from build123d import *

# Parameters (mm, degrees)
SKETCH1_W                = 90
SKETCH1_H                = 90
BOSS_EXTRUDE1_DEPTH      = 90
SKETCH4_W                = 40
SKETCH4_H                = 80
CUT_EXTRUDE3_DEPTH       = 90
SKETCH6_W                = 10
SKETCH6_H                = 2.5
CUT_EXTRUDE5_DEPTH       = 10
CUT_EXTRUDE6_DEPTH       = 90
CUT_EXTRUDE7_DEPTH       = 90
SKETCH10_W               = 2.5
SKETCH10_H               = 90
BOSS_EXTRUDE2_DEPTH      = 40
SKETCH11_W               = 2.5
SKETCH11_H               = 90
BOSS_EXTRUDE3_DEPTH      = 40
CUT_EXTRUDE10_DEPTH      = 37.5
SKETCH16_R               = 0.75
CUT_EXTRUDE12_DEPTH      = 1.5
CUT_EXTRUDE13_DEPTH      = 111.227038425
CUT_EXTRUDE13_DEPTH_BACK = 111.227038425
SKETCH17_R               = 0.75
SKETCH21_W               = 85
SKETCH21_H               = 2.5
CUT_EXTRUDE14_DEPTH      = 40
SKETCH22_W               = 85
SKETCH22_H               = 2.5
CUT_EXTRUDE15_DEPTH      = 40
SKETCH23_R               = 1.25
CUT_EXTRUDE16_DEPTH      = 1.5
SKETCH24_R               = 1.25
CUT_EXTRUDE17_DEPTH      = 1.5


with BuildPart() as part:
    # Sketch1 → Boss-Extrude1 (new body)
    with BuildSketch(Plane(origin=(0, 0, 0), x_dir=(1, 0, 0), z_dir=(0, 1, 0))):
        Rectangle(SKETCH1_W, SKETCH1_H)
    extrude(amount=BOSS_EXTRUDE1_DEPTH)

    # Sketch4 → Cut-Extrude3 (cut)
    with BuildSketch(Plane(origin=(0, 90, 0), x_dir=(1, 0, 0), z_dir=(0, 1, 0))):
        with Locations((-22.5, 0)):
            Rectangle(SKETCH4_W, SKETCH4_H)
        with Locations((22.5, 0)):
            Rectangle(SKETCH4_W, SKETCH4_H)
    extrude(amount=-CUT_EXTRUDE3_DEPTH, mode=Mode.SUBTRACT)

    # Sketch6 → Cut-Extrude5 (cut)
    with BuildSketch(Plane.XY.offset(45)):
        with Locations((7.5, 1.25)):
            Rectangle(SKETCH6_W, SKETCH6_H)
        with Locations((-7.5, 1.25)):
            Rectangle(SKETCH6_W, SKETCH6_H)
    extrude(amount=-CUT_EXTRUDE5_DEPTH, mode=Mode.SUBTRACT)

    # Sketch7 → Cut-Extrude6 (cut)
    with BuildSketch(Plane(origin=(0, 90, 0), x_dir=(1, 0, 0), z_dir=(0, 1, 0))):
        Polygon((42.5, 40), (42.5, 45), (45, 45), (45, -45), (42.5, -45), (42.5, -40), align=None)
    extrude(amount=-CUT_EXTRUDE6_DEPTH, mode=Mode.SUBTRACT)

    # Sketch8 → Cut-Extrude7 (cut)
    with BuildSketch(Plane(origin=(0, 90, 0), x_dir=(1, 0, 0), z_dir=(0, 1, 0))):
        Polygon((-42.5, 40), (-42.5, 45), (-45, 45), (-45, -45), (-42.5, -45), (-42.5, -42.5), align=None)
    extrude(amount=-CUT_EXTRUDE7_DEPTH, mode=Mode.SUBTRACT)

    # Sketch10 → Boss-Extrude2 (add)
    with BuildSketch(Plane.ZY.offset(2.5)):
        with Locations((-28.75, 45)):
            Rectangle(SKETCH10_W, SKETCH10_H)
    extrude(amount=BOSS_EXTRUDE2_DEPTH)

    # Sketch11 → Boss-Extrude3 (add)
    with BuildSketch(Plane(origin=(2.5, 0, 0), x_dir=(0, 0, -1), z_dir=(1, 0, 0))):
        with Locations((28.75, 45)):
            Rectangle(SKETCH11_W, SKETCH11_H)
    extrude(amount=BOSS_EXTRUDE3_DEPTH)

    # Sketch13 → Cut-Extrude10 (cut)
    with BuildSketch(Plane(origin=(42.5, 0, 0), x_dir=(0, 0, -1), z_dir=(1, 0, 0))):
        Polygon((40, 36), (40.5, 36), (40.5, 37), (41, 37), (41, 35), (40, 35), align=None)
        Polygon((29, 35), (30, 35), (30, 36), (29.5, 36), (29.5, 37), (29, 37), align=None)
    cut_extrude10 = extrude(amount=-CUT_EXTRUDE10_DEPTH, mode=Mode.SUBTRACT)

    # Mirror1: Cut-Extrude10 across plane
    add(cut_extrude10.mirror(Plane.ZY), mode=Mode.SUBTRACT)

    # Sketch16 → Cut-Extrude12 (cut)
    with BuildSketch(Plane(origin=(-12.5, 0, 0), x_dir=(0, 0, -1), z_dir=(1, 0, 0))):
        with Locations((-43.75, 1.2)):
            Circle(SKETCH16_R)
    extrude(amount=-CUT_EXTRUDE12_DEPTH, mode=Mode.SUBTRACT)

    # Sketch17 → Cut-Extrude13 (cut, two sides: drawn at the far end of the back side and taken through both)
    with BuildSketch(Plane.ZY.offset(2.5).offset(-CUT_EXTRUDE13_DEPTH_BACK)):
        with Locations(Location((43.75, 1.2, 0), (0, 0, 180))):
            Circle(SKETCH17_R)
    extrude(amount=CUT_EXTRUDE13_DEPTH + CUT_EXTRUDE13_DEPTH_BACK, mode=Mode.SUBTRACT)

    # Sketch21 → Cut-Extrude14 (cut)
    with BuildSketch(Plane(origin=(42.5, 0, 0), x_dir=(0, 0, -1), z_dir=(1, 0, 0))):
        with Locations((2.5, 1.25)):
            Rectangle(SKETCH21_W, SKETCH21_H)
    extrude(amount=-CUT_EXTRUDE14_DEPTH, mode=Mode.SUBTRACT)

    # Sketch22 → Cut-Extrude15 (cut)
    with BuildSketch(Plane.ZY.offset(42.5)):
        with Locations((-2.5, 1.25)):
            Rectangle(SKETCH22_W, SKETCH22_H)
    extrude(amount=-CUT_EXTRUDE15_DEPTH, mode=Mode.SUBTRACT)

    # Sketch23 → Cut-Extrude16 (cut)
    with BuildSketch(Plane(origin=(42.5, 0, 0), x_dir=(0, 0, -1), z_dir=(1, 0, 0))):
        with Locations((42.5, 87)):
            Circle(SKETCH23_R)
        with Locations(Location((42.5, 5.5, 0), (0, 0, 180))):
            Circle(SKETCH23_R)
    cut_extrude16 = extrude(amount=-CUT_EXTRUDE16_DEPTH, mode=Mode.SUBTRACT)

    # Sketch24 → Cut-Extrude17 (cut)
    with BuildSketch(Plane(origin=(42.5, 0, 0), x_dir=(0, 0, -1), z_dir=(1, 0, 0))):
        with Locations((-42.5, 87)):
            Circle(SKETCH24_R)
    cut_extrude17 = extrude(amount=-CUT_EXTRUDE17_DEPTH, mode=Mode.SUBTRACT)

    # Mirror2: Cut-Extrude16, Cut-Extrude17 across plane
    add(cut_extrude16.mirror(Plane.ZY), mode=Mode.SUBTRACT)
    add(cut_extrude17.mirror(Plane.ZY), mode=Mode.SUBTRACT)


solid = part.part
Work out the finished part from the listing and answer in its coordinate system (mm). A direction names the side the tool comes from. Coordinates: 2 decimals unless noted, no trailing zeros. Write each loop counter-clockwise with the first axis right and the second up, starting at its lowest first coordinate (ties: lowest second). Pieces come first, ordered by that corner, then holes.
1. The part is cut by section B-B, the plane x = -7. Write down the section's boundary in (y, z), and give its area (3 significant figures).
Results list:
outline: (2.5, -45) - (90, -45) - (90, -40) - (36, -40) - (36, -40.5) - (37, -40.5) - (37, -41) - (35, -41) - (35, -40) - (2.5, -40) - close; (2.5, -30) - (35, -30) - (35, -29) - (37, -29) - (37, -29.5) - (36, -29.5) - (36, -30) - (90, -30) - (90, -27.5) - (2.5, -27.5) - close; (2.5, 40) - (90, 40) - (90, 45) - (2.5, 45) - close
area: 1,090 mm2
2. Flat-ended cylindrical pins translate along their axes: pin 1 (1 mm diameter, centred on y = 52.5, z = -14, fed in from +X); pin 2 (1.5 mm diameter, centred on y = 9.5, z = 0.5, fed in from -X); pin 3 (5.5 mm diameter, centred on x = 16.5, z = -42.5, fed in from -Y). Find the tip coordinate at first contact, or state that the pin passes through.
Results list:
pin 1: stops at x = 2.5
pin 2: stops at x = -2.5
pin 3: stops at y = 2.5
3. Consider line 1 along Z through (x, y) = (17, 61); line 2 along Z through (x, y) = (41.45, 5.5); line 3 along Y through (x, z) = (41.65, 42.5). Determine where each line is inside the solid, lowest interval first.
Results list:
line 1: z = -45 to -40, -30 to -27.5, 40 to 45
line 2: z = -45 to -43.75, -41.25 to -40, -30 to -27.5, 40 to 45
line 3: y = 0 to 85.75, 88.25 to 90
4. For faces 1 (the flat face through (-22, 46, -27.5)), 2 (the flat face through (22, 46, 40)), 3 (the flat face through (41, 5, -43)), determine the directions among +Z, -Z, +X, -X, +Y, -Y from which every point of the face is accessible in a straight line to the end or side of a thin tool.
Results list:
face 1: -X, +Y, -Y
face 2: +X, +Y, -Y
face 3: +X
5. For a pull along Y with two mould halves and no side action, classify faces 4 (the cylindrical face through (-41.76, 6.26, -43.49)), 5 (the flat face through (42.5, 47, -43)), 6 (the flat face through (0, 0, -1)) as +Y half, -Y half, draft (parallel to the pull), parting line (faces both ways), or undercut.
Results list:
face 4: undercut
face 5: draft
face 6: -Y half
6. The part is cut by section D-D, the plane z = -42.5. Write down the section's boundary in (x, y).
Results list:
outline: (-42.5, 2.5) - (-2.5, 2.5) - (-2.5, 0) - (2.5, 0) - (2.5, 2.5) - (42.5, 2.5) - (42.5, 4.25) - (41, 4.25) - (41, 6.75) - (42.5, 6.75) - (42.5, 85.75) - (41, 85.75) - (41, 88.25) - (42.5, 88.25) - (42.5, 90) - (-42.5, 90) - (-42.5, 88.25) - (-41, 88.25) - (-41, 85.75) - (-42.5, 85.75) - (-42.5, 6.75) - (-41, 6.75) - (-41, 4.25) - (-42.5, 4.25) - close
7. The part is cut by section A-A, the plane x = -25.5. Write down the section's boundary in (y, z), and give its area (3 significant figures).
Results list:
outline: (0, 40) - (90, 40) - (90, 45) - (0, 45) - close; (2.5, -45) - (90, -45) - (90, -40) - (36, -40) - (36, -40.5) - (37, -40.5) - (37, -41) - (35, -41) - (35, -40) - (2.5, -40) - close; (2.5, -30) - (35, -30) - (35, -29) - (37, -29) - (37, -29.5) - (36, -29.5) - (36, -30) - (90, -30) - (90, -27.5) - (2.5, -27.5) - close; hole circle Ø1.5 at (1.2, 43.75)
area: 1,100 mm2
8. The part is cut by section C-C, the plane y = 57.5. Write down the section's boundary in (x, z).
Results list:
outline: (-42.5, -45) - (42.5, -45) - (42.5, -40) - (2.5, -40) - (2.5, -30) - (42.5, -30) - (42.5, -27.5) - (2.5, -27.5) - (2.5, 40) - (42.5, 40) - (42.5, 45) - (-42.5, 45) - (-42.5, 40) - (-2.5, 40) - (-2.5, -27.5) - (-42.5, -27.5) - (-42.5, -30) - (-2.5, -30) - (-2.5, -40) - (-42.5, -40) - close
